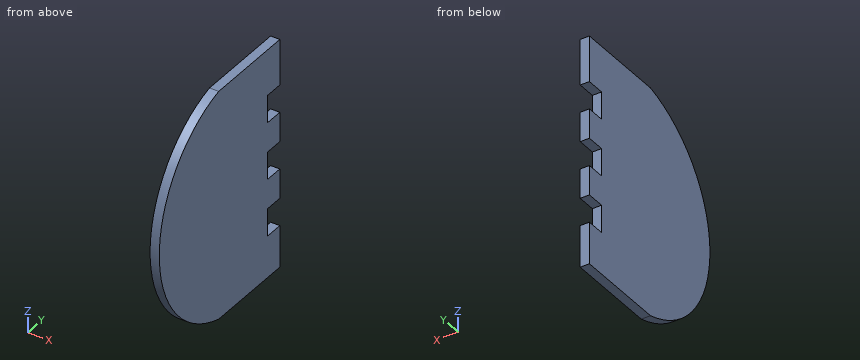
from build123d import *

# Parameters (mm, degrees)
BOSS_EXTRUDE2_DEPTH = 2.54
SKETCH3_W           = 2.54
SKETCH3_H           = 7.62
CUT_EXTRUDE2_DEPTH  = 5.08


with BuildPart() as part:
    # Sketch1 → Boss-Extrude2 (new body)
    with BuildSketch(Plane(origin=(0, 0, 0), x_dir=(0, 0, -1), z_dir=(1, 0, 0))):
        Polygon((-31.75, 33.376269743), (-31.75, 7.976269743), (31.75, 7.976269743), (31.75, 33.376269743), (0, 33.376269743), align=None)
        with BuildLine():
            ThreePointArc((31.75, 7.976269743), (0, -16.718131707), (-31.75, 7.976269743))
            Line((-31.75, 7.976269743), (31.75, 7.976269743))
        make_face()
    extrude(amount=BOSS_EXTRUDE2_DEPTH)

    # Sketch3 → Cut-Extrude2 (cut)
    with BuildSketch(Plane(origin=(0, 33.376269743, 0), x_dir=(1, 0, 0), z_dir=(0, 1, 0))):
        with Locations((1.27, -15.24)):
            Rectangle(SKETCH3_W, SKETCH3_H)
        with Locations((1.27, 0.557082085)):
            Rectangle(SKETCH3_W, SKETCH3_H)
        with Locations((1.27, 16.35416417)):
            Rectangle(SKETCH3_W, SKETCH3_H)
    extrude(amount=-CUT_EXTRUDE2_DEPTH, mode=Mode.SUBTRACT)


solid = part.part
CAD build for the part. Positions are in the model's coordinates, mm. Round coordinates to 2 decimals unless told otherwise and drop trailing zeros. Order: outer loops, then holes, each group sorted by start corner. A loop starts at its lowest first (then second) coordinate and runs counter-clockwise, first axis right, second up. Notation, with made-up numbers: M 87.5,20.25 L 141.5,20.25 A13 cw 141.5,26.25 Z; hole C 42,60.25 d7. An arc over 180 degrees is marked long. Use one line per item in the form item = value.
Q1. Flat gauge pin, fed straight in: P1, Ø5, axis at y = 5, z = 15, coming from the -X side. Where does the tip first touch, or does it go through?
Recorded:
P1 = 0
Q2. Saw through at B-B on x = 1.85. Give the cut face in (y, z), then the cut area to 3 significant figures.
Recorded:
outline = M 7.98,-31.75 L 33.38,-31.75 L 33.38,-20.16 L 28.3,-20.16 L 28.3,-12.54 L 33.38,-12.54 L 33.38,-4.37 L 28.3,-4.37 L 28.3,3.25 L 33.38,3.25 L 33.38,11.43 L 28.3,11.43 L 28.3,19.05 L 33.38,19.05 L 33.38,31.75 L 7.98,31.75 A32.76 ccw Z
area = 2,660 mm^2
Q3. Probe L1, parallel to Z at x = 2.3, y = 29; L2, parallel to Y at x = 0.9, z = 16; L3, parallel to Y at x = 0.8, z = 26. List the from-to ranges inside material, lowest first.
Recorded:
L1 = -31.75 to -20.16, -12.54 to -4.37, 3.25 to 11.43, 19.05 to 31.75
L2 = -12.54 to 28.3
L3 = -3.89 to 33.38
Q4. Saw through at D-D on y = 1.5. Give the cut face in (x, z).
Recorded:
outline = M 0,-29.35 L 2.54,-29.35 L 2.54,29.35 L 0,29.35 Z
Q5. Saw through at C-C on z = -19.5. Give the cut face in (x, y).
Recorded:
outline = M 0,-10.28 L 2.54,-10.28 L 2.54,28.3 L 0,28.3 Z
Q6. Saw through at A-A on y = 30. Give the cut face in (x, z).
Recorded:
outline = M 0,-31.75 L 2.54,-31.75 L 2.54,-20.16 L 0,-20.16 Z; M 0,-12.54 L 2.54,-12.54 L 2.54,-4.37 L 0,-4.37 Z; M 0,3.25 L 2.54,3.25 L 2.54,11.43 L 0,11.43 Z; M 0,19.05 L 2.54,19.05 L 2.54,31.75 L 0,31.75 Z
